Here's the drawing with two shaded views (mm, measured from the low corner). I have some questions. A direction names the side the tool comes from. Round coordinates to 2 decimals unless told otherwise and drop trailing zeros. Loops run counter-clockwise (first coordinate to the right, second up) from the corner with the lowest first, then second, coordinate; pieces in that order, holes last. Notation, with made-up numbers: (37, 87) -> (80, 87) arc R18 ccw to (80, 110) -> close; hole circle Ø11 at (34, -7). An arc over 180 degrees is marked (long way). Use a Markdown table: item, result.
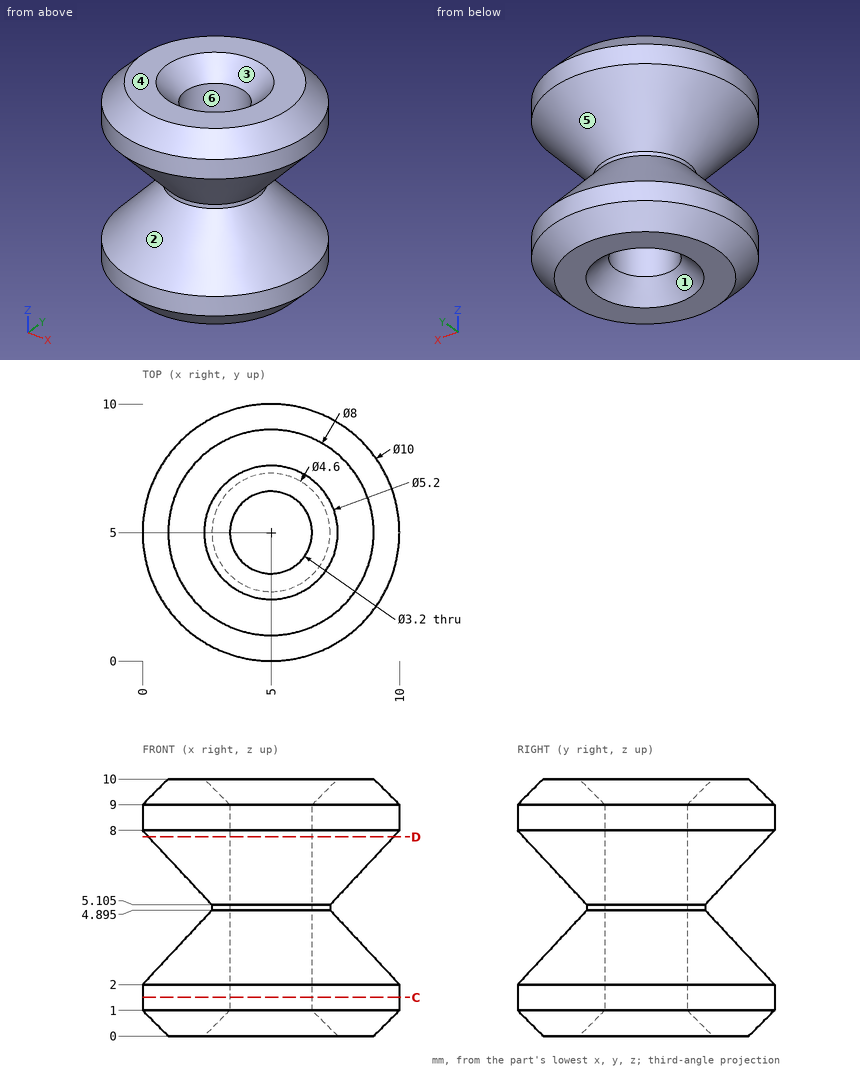
1. I want a section at C-C (z = 1.5). Please give me the cut outline in (x, y), plus the area to 3 significant figures.
Answer sheet:
| item | result |
|---|---|
| outline | circle Ø10 at (5, 5); hole circle Ø3.2 at (5, 5) |
| area | 70.5 mm² |
2. Will these pins go through, and if not, where does the flat tip stop? pin 1 Ø5 at (x, y) = (5, 5) entering from +Z; pin 2 Ø1 at (x, z) = (8, 5) entering from +Y; pin 3 Ø5 at (y, z) = (2, 8.5) entering from +X (1 decimal); pin 4 Ø2 at (x, z) = (2, 8) entering from +Y.
Answer sheet:
| item | result |
|---|---|
| pin 1 | stops at z = 9.9 |
| pin 2 | passes through |
| pin 3 | stops at x = 10 |
| pin 4 | stops at y = 9.58 |
3. If we mould it in two halves opening along Y, with no side actions, what happens to the marked faces 3, 4, 5 and 6? For each: +Y half, -Y half, draft (parallel to the pull), parting line (faces both ways), or undercut.
Answer sheet:
| item | result |
|---|---|
| face 3 | undercut |
| face 4 | draft |
| face 5 | parting line |
| face 6 | undercut |
4. I want a section at D-D (z = 7.75). Please give me the cut outline in (x, y).
Answer sheet:
| item | result |
|---|---|
| outline | circle Ø9.53 at (5, 5); hole circle Ø3.2 at (5, 5) |
5. Which directions (+Z, -Z, +X, -X, +Y, -Y) give clear straight access to the entire face, cutting with the end or side of a thin tool? Please do the marked faces 1 and 2.
Answer sheet:
| item | result |
|---|---|
| face 1 | -Z |
| face 2 | none |
6. I need wall thicknesses on line 1 (Y direction, x = 5, z = 5); line 2 (Y direction, x = 5, z = 4.5); line 3 (Z direction, x = 2.75, y = 7.25). Which ranges of each line are inside material? Lowest first, please.
Answer sheet:
| item | result |
|---|---|
| line 1 | y = 2.7 to 3.4, 6.6 to 7.3 |
| line 2 | y = 2.33 to 3.4, 6.6 to 7.67 |
| line 3 | z = 0 to 3.95, 6.05 to 10 |
